from build123d import *

# Parameters (mm, degrees)
BOSS_EXTRUDE1_DEPTH = 6.66
BOSS_EXTRUDE2_START = 10
SKETCH3_R           = 14.5
BOSS_EXTRUDE2_DEPTH = 10
BOSS_EXTRUDE3_START = -5
SKETCH5_W           = 27.34
SKETCH5_H           = 27.34
SKETCH5_W_2         = 21.34
SKETCH5_H_2         = 21.34
BOSS_EXTRUDE3_DEPTH = 83.34
SKETCH6_W           = 21.34
SKETCH6_H           = 21.34
BOSS_EXTRUDE4_DEPTH = 5
SKETCH8_W           = 21.34
SKETCH8_H           = 78.34
CUT_EXTRUDE1_DEPTH  = 5
SKETCH9_W           = 21.34
SKETCH9_H           = 3
CUT_EXTRUDE2_DEPTH  = 5
SKETCH10_W          = 27.34
SKETCH10_H          = 27.34
BOSS_EXTRUDE5_DEPTH = 3
SKETCH11_R          = 20.15
BOSS_EXTRUDE6_DEPTH = 12
SKETCH12_R          = 16.15
CUT_EXTRUDE3_DEPTH  = 10.5
SKETCH13_R          = 12.15
CUT_EXTRUDE4_DEPTH  = 0.5
BOSS_EXTRUDE7_START = 3
BOSS_EXTRUDE7_DEPTH = 3
SKETCH19_R          = 3.5
CUT_EXTRUDE5_DEPTH  = 112.972606961
SKETCH20_W          = 17.34
SKETCH20_H          = 20
CUT_EXTRUDE6_DEPTH  = 111.983314599
CUT_EXTRUDE7_DEPTH  = 111.983314599


with BuildPart() as part:
    # Sketch2 → Boss-Extrude1 (new body)
    with BuildSketch(Plane(origin=(0, 0, 0), x_dir=(1, 0, 0), z_dir=(0, 1, 0))):
        with BuildLine():
            Line((-4.257926427, 13.560157214), (-4.257926427, -1.390428058))
            ThreePointArc((-4.257926427, -1.390428058), (-0.281073012, 1.444552088), (1.242073573, 6.084864578))
            ThreePointArc((1.242073573, 6.084864578), (-0.281073012, 10.725177067), (-4.257926427, 13.560157214))
        make_face()
        with BuildLine():
            Line((-8.917926427, 13.560157214), (-8.917926427, -1.390428058))
            ThreePointArc((-8.917926427, -1.390428058), (-6.587926427, -1.745135422), (-4.257926427, -1.390428058))
            Line((-4.257926427, -1.390428058), (-4.257926427, 13.560157214))
            ThreePointArc((-4.257926427, 13.560157214), (-6.587926427, 13.914864578), (-8.917926427, 13.560157214))
        make_face()
        with BuildLine():
            Line((-8.917926427, -1.390428058), (-8.917926427, -4.245135422))
            Line((-8.917926427, -4.245135422), (-4.257926427, -4.245135422))
            Line((-4.257926427, -4.245135422), (-4.257926427, -1.390428058))
            ThreePointArc((-4.257926427, -1.390428058), (-6.587926427, -1.745135422), (-8.917926427, -1.390428058))
        make_face()
        with BuildLine():
            ThreePointArc((-8.917926427, 13.560157214), (-14.417926427, 6.084864578), (-8.917926427, -1.390428058))
            Line((-8.917926427, -1.390428058), (-8.917926427, 13.560157214))
        make_face()
        with BuildLine():
            Line((-8.917926427, 16.414864578), (-8.917926427, 13.560157214))
            ThreePointArc((-8.917926427, 13.560157214), (-6.587926427, 13.914864578), (-4.257926427, 13.560157214))
            Line((-4.257926427, 13.560157214), (-4.257926427, 16.414864578))
            Line((-4.257926427, 16.414864578), (-8.917926427, 16.414864578))
        make_face()
    extrude(amount=BOSS_EXTRUDE1_DEPTH)

    # Sketch3 → Boss-Extrude2 (add)
    # profile 1 of 3: a face of its own
    with BuildSketch(Plane.XZ.offset(BOSS_EXTRUDE2_START)):
        with Locations(Location((-6.587926427, -6.084864578, 0), (0, 0, 270))):
            Circle(SKETCH3_R)
        with BuildLine():
            ThreePointArc((-4.257926427, -13.560157214), (1.242073573, -6.084864578), (-4.257926427, 1.390428058))
            Line((-4.257926427, 1.390428058), (-4.257926427, 4.245135422))
            Line((-4.257926427, 4.245135422), (-8.917926427, 4.245135422))
            Line((-8.917926427, 4.245135422), (-8.917926427, 1.390428058))
            ThreePointArc((-8.917926427, 1.390428058), (-14.417926427, -6.084864578), (-8.917926427, -13.560157214))
            Line((-8.917926427, -13.560157214), (-8.917926427, -16.414864578))
            Line((-8.917926427, -16.414864578), (-4.257926427, -16.414864578))
            Line((-4.257926427, -16.414864578), (-4.257926427, -13.560157214))
        make_face(mode=Mode.SUBTRACT)
    # profile 2 of 3: a face of its own
    with BuildSketch(Plane.XZ.offset(BOSS_EXTRUDE2_START)):
        with BuildLine():
            Line((-4.257926427, 4.245135422), (-6.587926427, 4.245135422))
            Line((-6.587926427, 4.245135422), (-6.587926427, -16.414864578))
            Line((-6.587926427, -16.414864578), (-4.257926427, -16.414864578))
            Line((-4.257926427, -16.414864578), (-4.257926427, -13.560157214))
            ThreePointArc((-4.257926427, -13.560157214), (1.242073573, -6.084864578), (-4.257926427, 1.390428058))
            Line((-4.257926427, 1.390428058), (-4.257926427, 4.245135422))
        make_face()
    # profile 3 of 3: a face of its own
    with BuildSketch(Plane.XZ.offset(BOSS_EXTRUDE2_START)):
        with BuildLine():
            Line((-6.587926427, -16.414864578), (-6.587926427, 4.245135422))
            Line((-6.587926427, 4.245135422), (-8.917926427, 4.245135422))
            Line((-8.917926427, 4.245135422), (-8.917926427, 1.390428058))
            ThreePointArc((-8.917926427, 1.390428058), (-14.417926427, -6.084864578), (-8.917926427, -13.560157214))
            Line((-8.917926427, -13.560157214), (-8.917926427, -16.414864578))
            Line((-8.917926427, -16.414864578), (-6.587926427, -16.414864578))
        make_face()
    extrude(amount=-BOSS_EXTRUDE2_DEPTH)

    # Sketch5 → Boss-Extrude3 (add)
    with BuildSketch(Plane.XZ.offset(10).offset(BOSS_EXTRUDE3_START)):
        with Locations((-6.587926427, -6.084864578)):
            Rectangle(SKETCH5_W, SKETCH5_H)
        with Locations((-6.587926427, -6.084864578)):
            Rectangle(SKETCH5_W_2, SKETCH5_H_2, mode=Mode.SUBTRACT)
    extrude(amount=BOSS_EXTRUDE3_DEPTH)

    # Sketch6 → Boss-Extrude4 (add)
    with BuildSketch(Plane.XZ.offset(10)):
        with Locations((-6.587926427, -6.084864578)):
            Rectangle(SKETCH6_W, SKETCH6_H)
    extrude(amount=-BOSS_EXTRUDE4_DEPTH)

    # Sketch8 → Cut-Extrude1 (cut)
    with BuildSketch(Plane.ZY.offset(20.257926427)):
        with Locations((-6.084864578, -49.17)):
            Rectangle(SKETCH8_W, SKETCH8_H)
    extrude(amount=-CUT_EXTRUDE1_DEPTH, mode=Mode.SUBTRACT)

    # Sketch9 → Cut-Extrude2 (cut)
    with BuildSketch(Plane.ZY.offset(-4.082073573)):
        with Locations((-6.084864578, -11.5)):
            Rectangle(SKETCH9_W, SKETCH9_H)
    extrude(amount=-CUT_EXTRUDE2_DEPTH, mode=Mode.SUBTRACT)

    # Sketch10 → Boss-Extrude5 (add)
    with BuildSketch(Plane.XZ.offset(88.34)):
        with Locations((-6.587926427, -6.084864578)):
            Rectangle(SKETCH10_W, SKETCH10_H)
    extrude(amount=BOSS_EXTRUDE5_DEPTH)

    # Sketch11 → Boss-Extrude6 (add)
    with BuildSketch(Plane(origin=(0, -91.34, 0), x_dir=(-1, 0, 0), z_dir=(0, -1, 0))):
        with Locations(Location((6.587926427, 6.084864578, 0), (0, 0, 90))):
            Circle(SKETCH11_R)
    extrude(amount=BOSS_EXTRUDE6_DEPTH)

    # Sketch12 → Cut-Extrude3 (cut)
    with BuildSketch(Plane.XZ.offset(103.34)):
        with Locations(Location((-6.587926427, -6.084864578, 0), (0, 0, 270))):
            Circle(SKETCH12_R)
    extrude(amount=-CUT_EXTRUDE3_DEPTH, mode=Mode.SUBTRACT)

    # Sketch13 → Cut-Extrude4 (cut)
    with BuildSketch(Plane.XZ.offset(92.84)):
        with Locations(Location((-6.587926427, -6.084864578, 0), (0, 0, 270))):
            Circle(SKETCH13_R)
    extrude(amount=-CUT_EXTRUDE4_DEPTH, mode=Mode.SUBTRACT)

    # Sketch14 → Boss-Extrude7 (add)
    with BuildSketch(Plane(origin=(0, -91.34, 0), x_dir=(1, 0, 0), z_dir=(0, 1, 0)).offset(BOSS_EXTRUDE7_START)):
        with BuildLine():
            Line((-6.587926427, -7.585135422), (-6.587926427, -14.065135422))
            ThreePointArc((-6.587926427, -14.065135422), (7.660275213, -8.163337063), (13.562073573, 6.084864578))
            ThreePointArc((13.562073573, 6.084864578), (7.660275213, 20.333066219), (-6.587926427, 26.234864578))
            Line((-6.587926427, 26.234864578), (-6.587926427, 19.754864578))
            Line((-6.587926427, 19.754864578), (7.082073573, 19.754864578))
            Line((7.082073573, 19.754864578), (7.082073573, -7.585135422))
            Line((7.082073573, -7.585135422), (-6.587926427, -7.585135422))
        make_face()
        with BuildLine():
            ThreePointArc((-6.587926427, 26.234864578), (-26.737926427, 6.084864578), (-6.587926427, -14.065135422))
            Line((-6.587926427, -14.065135422), (-6.587926427, -7.585135422))
            Line((-6.587926427, -7.585135422), (-20.257926427, -7.585135422))
            Line((-20.257926427, -7.585135422), (-20.257926427, 19.754864578))
            Line((-20.257926427, 19.754864578), (-6.587926427, 19.754864578))
            Line((-6.587926427, 19.754864578), (-6.587926427, 26.234864578))
        make_face()
    extrude(amount=-BOSS_EXTRUDE7_DEPTH)

    # Sketch19 → Cut-Extrude5 (cut, through all)
    with BuildSketch(Plane.XY.offset(7.585135422)):
        with Locations((-6.587926427, -49.17)):
            Circle(SKETCH19_R)
    extrude(amount=-CUT_EXTRUDE5_DEPTH, mode=Mode.SUBTRACT)

    # Sketch20 → Cut-Extrude6 (cut, through all)
    with BuildSketch(Plane.ZY.offset(-4.082073573)):
        with Locations((-6.084864578, -25)):
            Rectangle(SKETCH20_W, SKETCH20_H)
    extrude(amount=-CUT_EXTRUDE6_DEPTH, mode=Mode.SUBTRACT)

    # Sketch21 → Cut-Extrude7 (cut, through all)
    with BuildSketch(Plane.ZY.offset(-4.082073573)):
        Polygon((-14.754864578, -15), (-16.754864578, -13), (4.585135422, -13), (2.585135422, -15), align=None)
    extrude(amount=-CUT_EXTRUDE7_DEPTH, mode=Mode.SUBTRACT)


solid = part.part
Verification items for the finished model (mm, model axes). A direction names the side the tool comes from. Round coordinates to 2 decimals unless told otherwise and drop trailing zeros. Loops run counter-clockwise (first coordinate to the right, second up) from the corner with the lowest first, then second, coordinate; pieces in that order, holes last. Notation, with made-up numbers: M 59,15.5 L 83,15.5 A30 ccw 83,46.5 Z; hole C 58.5,61 d11. An arc over 180 degrees is marked long. Write each question's results on one line, items separated by ' | '.
1) Gauge pin test, flat ends, axial feed: P1, Ø2.5, axis at y = 3.5, z = -14.5, coming from the -X side; P2, Ø8, axis at x = -3.5, y = -36, coming from the -Z side; P3, Ø3, axis at y = 3, z = -14.5, coming from the +X side; P4, Ø10, axis at x = -3.5, y = -87, coming from the -Z side. Record the tip position at first contact, or that the pin passes through.
Checks:
P1: stops at x = -9.75 | P2: stops at z = -19.75 | P3: stops at x = -2.92 | P4: stops at z = -26.23
2) Section check D-D on z = -4. Record the boundary of the cut face in (x, y).
Checks:
outline: M -26.63,-103.34 L -22.6,-103.34 L -22.6,-92.84 L -18.56,-92.84 L -18.56,-92.34 L 5.38,-92.34 L 5.38,-92.84 L 9.43,-92.84 L 9.43,-103.34 L 13.45,-103.34 L 13.45,-88.34 L 7.08,-88.34 L 7.08,-35 L 4.08,-35 L 4.08,-88.34 L -26.63,-88.34 Z; M -20.94,-10 L 7.76,-10 L 7.76,0 L 0.96,0 L 0.96,6.66 L -14.14,6.66 L -14.14,0 L -20.94,0 Z
3) Mould release check, pull along Y, two halves, no side actions. Record for faces 1 (the flat face through (7.082, -55, -6)), 2 (the flat face through (-6, -92.34, -6)), 3 (the cylindrical face through (-16.415, -98.164, 6.731)), 4 (the flat face through (-18, -5, 5)): released by +Y, released by -Y, zero draft, split by the parting line, or undercut.
Checks:
face 1: undercut | face 2: released by -Y | face 3: zero draft | face 4: released by +Y
4) Scan lines: L1, parallel to Z at x = -17, y = -20.5; L2, parallel to Y at x = -13, z = -1.5; L3, parallel to Y at x = -19, z = -1.5. Record each from-to range of solid material in increasing order. Write a range as from..to.
Checks:
L1: z = -19.75..-16.75, 4.59..7.59 | L2: y = -92.34..-88.34, -10..0 | L3: y = -92.84..-88.34, -10..0
5) Section check A-A on y = -49.17. Record the boundary of the cut face in (x, z).
Checks:
outline: M -20.26,-19.75 L -10.09,-19.75 L -10.09,-16.75 L -20.26,-16.75 Z; M -20.26,4.59 L -10.09,4.59 L -10.09,7.59 L -20.26,7.59 Z; M -3.09,-19.75 L 7.08,-19.75 L 7.08,7.59 L -3.09,7.59 L -3.09,4.59 L 4.08,4.59 L 4.08,-16.75 L -3.09,-16.75 Z
6) Section check B-B on y = -7. Record the boundary of the cut face in (x, z).
Checks:
outline: M -20.26,-19.75 L -11.42,-19.75 A14.5 ccw -1.75,-19.75 L 7.08,-19.75 L 7.08,-10.92 A14.5 ccw 7.08,-1.25 L 7.08,7.59 L -1.75,7.59 A14.5 ccw -11.42,7.59 L -20.26,7.59 L -20.26,-1.25 A14.5 ccw -20.26,-10.92 Z
7) Section check C-C on x = 3. Record the boundary of the cut face in (y, z), then the cut area to 3 significant figures.
Checks:
outline: M -103.34,-23.81 L -88.34,-23.81 L -88.34,-19.75 L -5,-19.75 L -5,-16.96 L 0,-16.96 L 0,4.79 L -5,4.79 L -5,7.59 L -88.34,7.59 L -88.34,11.64 L -103.34,11.64 L -103.34,6.91 L -92.84,6.91 L -92.84,1.38 L -92.34,1.38 L -92.34,-13.55 L -92.84,-13.55 L -92.84,-19.08 L -103.34,-19.08 Z; hole M -88.34,-16.75 L -10,-16.75 L -10,4.59 L -88.34,4.59 Z | area: 967 mm2
8) Access from +Z, -Z, +X, -X, +Y, -Y to the whole of each face (thin tool, end or side, straight path). Record for faces 5 (the flat face through (-8.918, 3, 3)), 6 (the flat face through (5.5, -92.84, -8.4)), 7 (the flat face through (-6, -10, -6)).
Checks:
face 5: +Z, -X, +Y | face 6: -Y | face 7: +X, -X
